Work out the finished part from the listing and answer in its coordinate system (mm). Round coordinates to 2 decimals unless told otherwise and drop trailing zeros. Write each loop counter-clockwise with the first axis right and the second up, starting at its lowest first coordinate (ties: lowest second). Pieces come first, ordered by that corner, then holes. Notation, with made-up numbers: M 24,65.5 L 65,65.5 A35 ccw 65,101.5 Z; hole C 52,87 d9. An arc over 180 degrees is marked long. Answer in a Markdown table with one row per item.
```python
from build123d import *

# Parameters (mm, degrees)
F0_R     = 35.71875
F0_R_2   = 2.54
F1_DEPTH = 3.175


# Not quite as in the source:
# - a length typed as a fraction of an inch, garbled in the dataset ("3 / 203.2 mm" for 3/8 in), is restored


with BuildPart() as f1:
    # F0 (on Right) → F1 (new body)
    with BuildSketch(Plane.YZ):
        Circle(F0_R)
        with BuildLine():
            ThreePointArc((0, -31.75), (-12.1501989776, -29.3331751572), (-22.4506403027, -22.4506403027))
            Line((-22.4506403027, -22.4506403027), (-8.9802561211, -8.9802561211))
            ThreePointArc((-8.9802561211, -8.9802561211), (-4.860079591, -11.7332700629), (0, -12.7))
            Line((0, -12.7), (0, -31.75))
        make_face(mode=Mode.SUBTRACT)
        with BuildLine():
            ThreePointArc((8.9802561211, -8.9802561211), (11.7332700629, -4.860079591), (12.7, 0))
            Line((12.7, 0), (31.75, 0))
            ThreePointArc((31.75, 0), (29.3331751572, -12.1501989776), (22.4506403027, -22.4506403027))
            Line((22.4506403027, -22.4506403027), (8.9802561211, -8.9802561211))
        make_face(mode=Mode.SUBTRACT)
        with BuildLine():
            ThreePointArc((-8.9802561211, 8.9802561211), (-11.7332700629, 4.860079591), (-12.7, 0))
            Line((-12.7, 0), (-31.75, 0))
            ThreePointArc((-31.75, 0), (-29.3331751572, 12.1501989776), (-22.4506403027, 22.4506403027))
            Line((-22.4506403027, 22.4506403027), (-8.9802561211, 8.9802561211))
        make_face(mode=Mode.SUBTRACT)
        Circle(F0_R_2, mode=Mode.SUBTRACT)
        with BuildLine():
            ThreePointArc((8.9802561211, 8.9802561211), (4.860079591, 11.7332700629), (0, 12.7))
            Line((0, 12.7), (0, 31.75))
            ThreePointArc((0, 31.75), (12.1501989776, 29.3331751572), (22.4506403027, 22.4506403027))
            Line((22.4506403027, 22.4506403027), (8.9802561211, 8.9802561211))
        make_face(mode=Mode.SUBTRACT)
    extrude(amount=F1_DEPTH)


solid = f1.part
```
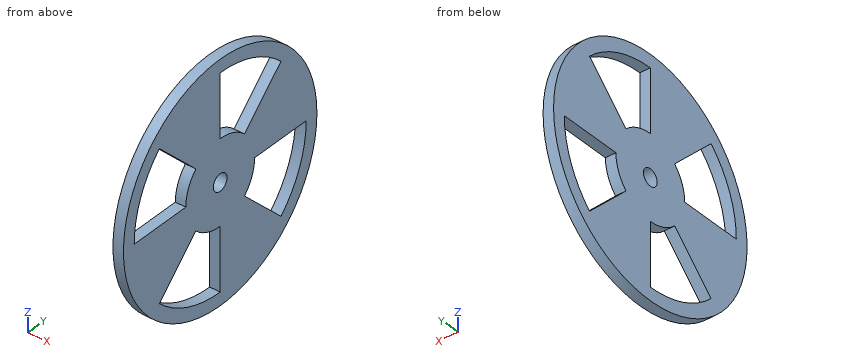
1. The part is cut by section A-A (x = 1). Determine the outline of the cut face in (y, z), plus the area to 3 significant figures.
Calculated:
| item | result |
|---|---|
| outline | C 0,0 d71.44; hole M -31.75,0 L -12.7,0 A12.7 cw -8.98,8.98 L -22.45,22.45 A31.75 ccw Z; hole M -22.45,-22.45 A31.75 ccw 0,-31.75 L 0,-12.7 A12.7 cw -8.98,-8.98 Z; hole C 0,0 d5.08; hole M 0,12.7 A12.7 cw 8.98,8.98 L 22.45,22.45 A31.75 ccw 0,31.75 Z; hole M 8.98,-8.98 L 22.45,-22.45 A31.75 ccw 31.75,0 L 12.7,0 A12.7 cw Z |
| area | 2,660 mm² |
2. The part is cut by section B-B (y = 10.5). Determine the outline of the cut face in (x, z) (3 decimals).
Calculated:
| item | result |
|---|---|
| outline | M 0,-34.141 L 3.175,-34.141 L 3.175,-10.5 L 0,-10.5 Z; M 0,-7.144 L 3.175,-7.144 L 3.175,10.5 L 0,10.5 Z; M 0,29.964 L 3.175,29.964 L 3.175,34.141 L 0,34.141 Z |
3. The part is cut by section C-C (z = -11). Determine the outline of the cut face in (x, y) (3 decimals), plus the area to 3 significant figures.
Calculated:
| item | result |
|---|---|
| outline | M 0,-33.983 L 3.175,-33.983 L 3.175,-11 L 0,-11 Z; M 0,-6.347 L 3.175,-6.347 L 3.175,11 L 0,11 Z; M 0,29.784 L 3.175,29.784 L 3.175,33.983 L 0,33.983 Z |
| area | 141 mm² |
4. Given pin 1 (1.5 mm diameter, centred on y = -6.5, z = -11.5, fed in from +X) (3 decimals); pin 2 (1 mm diameter, centred on x = 1, z = 24, fed in from +Y); pin 3 (3 mm diameter, centred on y = 0, z = 0, fed in from -X); pin 4 (1.6 mm diameter, centred on x = 2, z = -24, fed in from -Y), each flat-ended and moving along its own axis, determine where each tip first touches the part or whether it passes through.
Calculated:
| item | result |
|---|---|
| pin 1 | stops at x = 3.175 |
| pin 2 | stops at y = 26.9 |
| pin 3 | passes through |
| pin 4 | stops at y = -27.16 |
5. Consider line 1 along Y through (x, z) = (1.9, 14.5); line 2 along Y through (x, z) = (1.7, 20.5); line 3 along Z through (x, y) = (0.85, 2). Determine where each line is inside the solid, lowest interval first. Write a range as from..to.
Calculated:
| item | result |
|---|---|
| line 1 | y = -32.64..-28.25, -14.5..0, 14.5..32.64 |
| line 2 | y = -29.25..-24.24, -20.5..0, 20.5..29.25 |
| line 3 | z = -35.66..-1.57, 1.57..12.54, 31.69..35.66 |
6. The part is cut by section D-D (y = -8). Determine the outline of the cut face in (x, z) (3 decimals).
Calculated:
| item | result |
|---|---|
| outline | M 0,-34.811 L 3.175,-34.811 L 3.175,-30.726 L 0,-30.726 Z; M 0,-9.864 L 3.175,-9.864 L 3.175,34.811 L 0,34.811 Z |
